Can you work these out from the drawing? Everything is in mm from the part's minimum corner. A direction names the side the tool comes from. Give positions to 0.01 mm unless a question says otherwise; leave off trailing zeros. Order: outer loops, then holes, each group sorted by start corner. A loop starts at its lowest first (then second) coordinate and runs counter-clockwise, first axis right, second up. Notation, with made-up numbers: M -34,45.5 L -3,45.5 A27 ccw -3,65.5 Z; hole C 57,84 d11. An arc over 180 degrees is marked long. Answer in a Markdown table with one row per item. Add a question column.
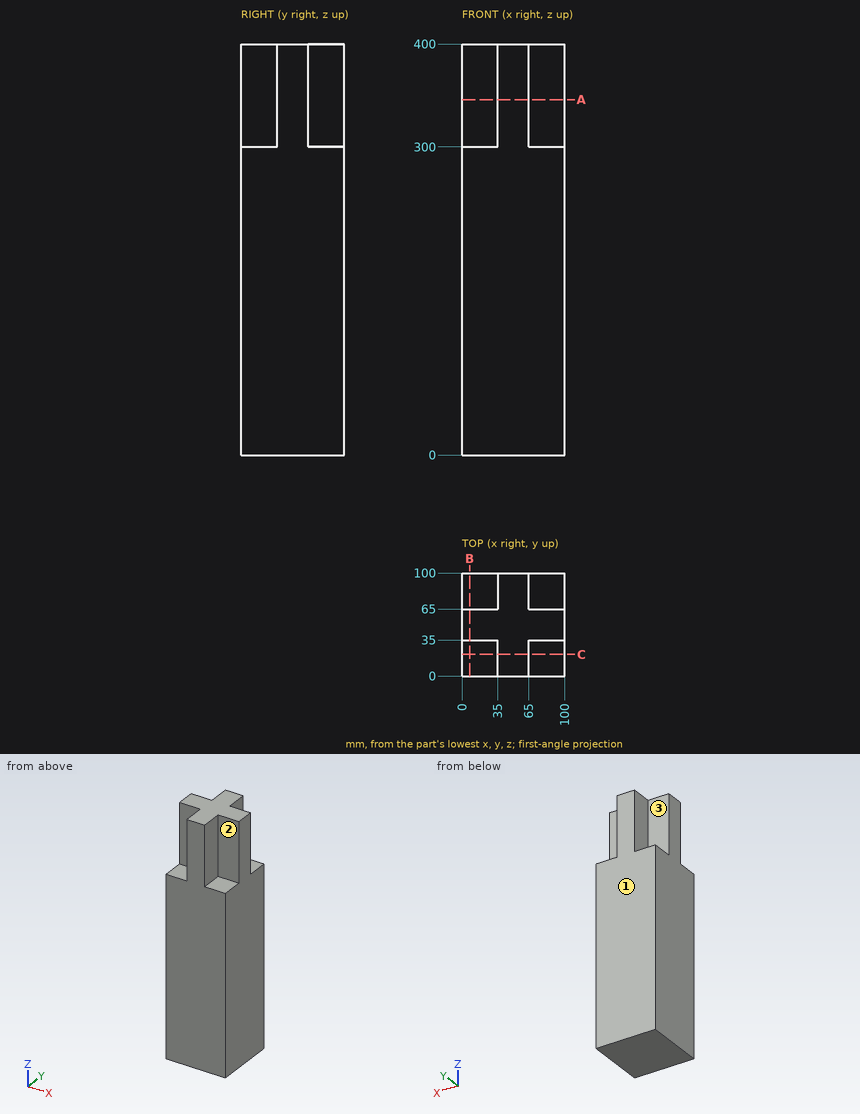
1. Will these pins go through, and if not, where does the flat tip stop? P1, Ø17.5, axis at y = 14, z = 337.5, coming from the -X side; P2, Ø17.5, axis at x = 16.5, z = 361, coming from the +Y side; P3, Ø17.5, axis at y = 82, z = 335, coming from the +X side.
2. If I drill on line 1 along Z through (x, y) = (19, 5.5); line 2 along X through (y, z) = (82, 313.5), over which ranges is the centre line in solid material (lowest first)? Write a range as [from, to].
3. Suppose I cut it at B-B on x = 7.5. List the corners of the cut face in (y, z) for me, plus the area to 3 significant figures.
4. For the marked faces 1, 2 and 3, which set-ups out of +Z, -Z, +X, -X, +Y, -Y let a thin tool reach every point of the face, with its end or its side?
5. Suppose I cut it at A-A on z = 346. List the corners of the cut face in (x, y) for me, plus the area to 3 significant figures.
Findings below:
| question | item | result |
|---|---|---|
| 1 | P1 | x = 35 |
| 1 | P2 | y = 65 |
| 1 | P3 | x = 65 |
| 2 | line 1 | [0, 300] |
| 2 | line 2 | [35, 65] |
| 3 | outline | M 0,0 L 100,0 L 100,300 L 65,300 L 65,400 L 35,400 L 35,300 L 0,300 Z |
| 3 | area | 33,000 mm2 |
| 4 | face 1 | +Z, -Z, +X, -X, +Y |
| 4 | face 2 | +Z, +X, -Y |
| 4 | face 3 | +Z, -X, +Y |
| 5 | outline | M 0,35 L 35,35 L 35,0 L 65,0 L 65,35 L 100,35 L 100,65 L 65,65 L 65,100 L 35,100 L 35,65 L 0,65 Z |
| 5 | area | 5,100 mm2 |
